```python
from build123d import *

# Parameters (mm, degrees)
SKETCH1_R           = 2
SKETCH1_R_2         = 2.5
SKETCH1_R_3         = 1.5
BOSS_EXTRUDE3_DEPTH = 2.5
SKETCH1_5_R         = 2
SKETCH1_5_R_2       = 1.5
CUT_EXTRUDE1_DEPTH  = 0.333333333


with BuildPart() as part:
    # Sketch1 → Boss-Extrude3 (new body)
    with BuildSketch(Plane(origin=(0, 0, 0), x_dir=(1, 0, 0), z_dir=(0, 1, 0))):
        with BuildLine():
            ThreePointArc((5, 2.5), (4.267766953, 0.732233047), (2.5, 0))
            Line((2.5, 0), (12.5, 0))
            ThreePointArc((12.5, 0), (10, 2.5), (12.5, 5))
            Line((12.5, 5), (2.5, 5))
            ThreePointArc((2.5, 5), (4.267766953, 4.267766953), (5, 2.5))
        make_face()
        with Locations((7.5, 2.5)):
            Circle(SKETCH1_R, mode=Mode.SUBTRACT)
        with Locations((2.5, 2.5)):
            Circle(SKETCH1_R_2)
        with Locations((2.5, 2.5)):
            Circle(SKETCH1_R, mode=Mode.SUBTRACT)
        with Locations((2.5, 2.5)):
            Circle(SKETCH1_R)
        with Locations(Location((2.5, 2.5, 0), (0, 0, 270))):
            Circle(SKETCH1_R_3, mode=Mode.SUBTRACT)
        with Locations((12.5, 2.5)):
            Circle(SKETCH1_R_2)
        with Locations((12.5, 2.5)):
            Circle(SKETCH1_R, mode=Mode.SUBTRACT)
        with Locations((12.5, 2.5)):
            Circle(SKETCH1_R)
        with Locations(Location((12.5, 2.5, 0), (0, 0, 270))):
            Circle(SKETCH1_R_3, mode=Mode.SUBTRACT)
        with Locations((7.5, 2.5)):
            Circle(SKETCH1_R)
        with Locations(Location((7.5, 2.5, 0), (0, 0, 270))):
            Circle(SKETCH1_R_3, mode=Mode.SUBTRACT)
    boss_extrude3 = extrude(amount=BOSS_EXTRUDE3_DEPTH)

    # Sketch1_5 → Cut-Extrude1 (cut)
    with BuildSketch(Plane(origin=(0, 0, 0), x_dir=(1, 0, 0), z_dir=(0, 1, 0))):
        with Locations(Location((12.5, 2.5, 0), (0, 0, 270))):
            Circle(SKETCH1_5_R)
        with Locations(Location((12.5, 2.5, 0), (0, 0, 270))):
            Circle(SKETCH1_5_R_2, mode=Mode.SUBTRACT)
        with Locations(Location((7.5, 2.5, 0), (0, 0, 270))):
            Circle(SKETCH1_5_R)
        with Locations(Location((7.5, 2.5, 0), (0, 0, 270))):
            Circle(SKETCH1_5_R_2, mode=Mode.SUBTRACT)
        with Locations(Location((2.5, 2.5, 0), (0, 0, 270))):
            Circle(SKETCH1_5_R)
        with Locations(Location((2.5, 2.5, 0), (0, 0, 270))):
            Circle(SKETCH1_5_R_2, mode=Mode.SUBTRACT)
    cut_extrude1 = extrude(amount=CUT_EXTRUDE1_DEPTH, mode=Mode.SUBTRACT)

    # Mirror2: Boss-Extrude3, Cut-Extrude1 across plane
    add(boss_extrude3.mirror(Plane.ZX.offset(2.5)))
    add(cut_extrude1.mirror(Plane.ZX.offset(2.5)), mode=Mode.SUBTRACT)


solid = part.part
```
Work out the finished part from the listing and answer in its coordinate system (mm). A direction names the side the tool comes from. Give positions to 0.01 mm unless a question says otherwise; leave off trailing zeros. Order: outer loops, then holes, each group sorted by start corner. A loop starts at its lowest first (then second) coordinate and runs counter-clockwise, first axis right, second up.
1. The mould has two halves that part along Z. Classify faces 4 (the cylindrical face through (0.548, 4.836, -2.934)), 5 (the flat face through (5.7, 5, -4.2)), 6 (the flat face through (7, 3, 0)): released by +Z, released by -Z, zero draft, split by the parting line, or undercut.
Result sheet:
face 4: undercut
face 5: zero draft
face 6: released by +Z
2. For faces 1 (the cylindrical face through (15, 2.5, -2.4)), 2 (the cylindrical face through (14.483, 4.836, -2.76)), 3 (the cylindrical face through (9.483, 0.164, -2.76)), determine the directions among +Z, -Z, +X, -X, +Y, -Y from which every point of the face is accessible in a straight line to the end or side of a thin tool.
Result sheet:
face 1: +X, +Y, -Y
face 2: +Y
face 3: -Y
3. Straight lines are drawn through the part: L1, parallel to X at y = 2.2, z = -2.5; L2, parallel to X at y = 0.15, z = -2.5; L3, parallel to Z at x = 13.5, y = 1.1. For each, find the intervals that lie inside material, in ascending order.
Result sheet:
L1: x = 0 to 1, 4 to 6, 9 to 11, 14 to 15
L2: x = 0 to 0.5, 4.5 to 5.5, 9.5 to 10.5, 14.5 to 15
L3: z = -4.79 to -3.62, -1.38 to -0.21
4. Section B-B, the plane y = 3.1 is taken. Determine the outline of the cut face in (x, z), and give its area (3 significant figures).
Result sheet:
outline: (2.5, -5) - (12.5, -5) arc R2.5 ccw to (12.5, 0) - (2.5, 0) arc R2.5 ccw to start; hole circle Ø3 at (2.5, -2.5); hole circle Ø3 at (7.5, -2.5); hole circle Ø3 at (12.5, -2.5)
area: 48.4 mm2
5. This flat-tipped pin is pushed along its axis until it touches: P1, Ø1.2, axis at x = 13, z = -2.5, coming from the -Y side. Where does it stop, or does it pass through?
Result sheet:
P1: passes through
6. Section A-A, the plane x = 7.5 is taken. Determine the outline of the cut face in (y, z).
Result sheet:
outline: (0, -5) - (5, -5) - (5, -4.5) - (4.67, -4.5) - (4.67, -4) - (0.33, -4) - (0.33, -4.5) - (0, -4.5) - close; (0, -0.5) - (0.33, -0.5) - (0.33, -1) - (4.67, -1) - (4.67, -0.5) - (5, -0.5) - (5, 0) - (0, 0) - close
7. Section D-D, the plane x = 12 is taken. Determine the outline of the cut face in (y, z).
Result sheet:
outline: (0, -5) - (5, -5) - (5, -4.44) - (4.67, -4.44) - (4.67, -3.91) - (0.33, -3.91) - (0.33, -4.44) - (0, -4.44) - close; (0, -0.56) - (0.33, -0.56) - (0.33, -1.09) - (4.67, -1.09) - (4.67, -0.56) - (5, -0.56) - (5, 0) - (0, 0) - close
8. Section C-C, the plane z = -0.65 is taken. Determine the outline of the cut face in (x, y), and give its area (3 significant figures).
Result sheet:
outline: (0.82, 0) - (1.74, 0) - (1.74, 0.33) - (3.26, 0.33) - (3.26, 0) - (6.74, 0) - (6.74, 0.33) - (8.26, 0.33) - (8.26, 0) - (11.74, 0) - (11.74, 0.33) - (13.26, 0.33) - (13.26, 0) - (14.18, 0) - (14.18, 5) - (13.26, 5) - (13.26, 4.67) - (11.74, 4.67) - (11.74, 5) - (8.26, 5) - (8.26, 4.67) - (6.74, 4.67) - (6.74, 5) - (3.26, 5) - (3.26, 4.67) - (1.74, 4.67) - (1.74, 5) - (0.82, 5) - close
area: 63.8 mm2
